The listing builds one solid part. Answer for the finished solid, in the listing's coordinates (mm). A direction names the side the tool comes from. Round coordinates to 2 decimals unless told otherwise and drop trailing zeros. Loops run counter-clockwise (first coordinate to the right, second up) from the corner with the lowest first, then second, coordinate; pieces in that order, holes last. Notation, with made-up numbers: (-33.75, 20.25) -> (24.25, 20.25) arc R12 cw to (24.25, 31.25) -> close; hole circle Ø7 at (-12, -1). An arc over 180 degrees is marked (long way). Write each question's results on one line, items separated by ' | '. Start each with the question number.
(1) The part is cut by section D-D (x = -9.75). Determine the outline of the cut face in (y, z), plus the area to 3 significant figures.
(2) The part is cut by section B-B (x = 0). Determine the outline of the cut face in (y, z).
(3) The part is cut by section C-C (z = 16.75). Determine the outline of the cut face in (x, y), plus the area to 3 significant figures.
(4) Straight lines are drawn through the part: probe 1 along Y at (x, z) = (0.25, 17.75); probe 2 along Z at (x, y) = (2.5, 5.25); probe 3 along Y at (x, z) = (-1.75, 25.25). For each, find the intervals that lie inside material, in ascending order.
(5) Flat-ended cylindrical pins translate along their axes: pin 1 (5 mm diameter, centred on x = -4, y = 5.5, fed in from +Z); pin 2 (1.5 mm diameter, centred on y = -13, z = 9, fed in from +X); pin 3 (10 mm diameter, centred on y = -1.5, z = 16, fed in from -X); pin 4 (6 mm diameter, centred on y = -8.5, z = 20, fed in from +X). Find the tip coordinate at first contact, or state that the pin passes through.
(6) The part is cut by section A-A (y = -4). Determine the outline of the cut face in (x, z), plus the area to 3 significant figures.
(7) Determine the mould class of faces 1 (the face through (-10.316, 3.91, 1.521)), 2 (the face through (-3, -7, 0)), 3 (the face through (11.693, -3.933, 1.479)) for opening direction Y: released by +Y, released by -Y, zero draft, split by the parting line, or undercut.
(8) For faces 4 (the face through (6, 2, 3)), 5 (the face through (0.33, 4.67, 1.48)), determine the directions among +Z, -Z, +X, -X, +Y, -Y from which every point of the face is accessible in a straight line to the end or side of a thin tool.
```python
from build123d import *

# Parameters (mm, degrees)
CROQUIS2_R            = 1.530907885
CORTAR_EXTRUIR1_DEPTH = 10


with BuildPart() as part:
    # Croquis1 → Revolución1 (revolve)
    with BuildSketch(Plane(origin=(0, 0, 0), x_dir=(0, 0, -1), z_dir=(1, 0, 0)), mode=Mode.PRIVATE) as revoluci_n1_sk:
        Polygon((0, 0), (0, 9), (-3, 9), (-3, 3), (-30, 3), (-30, 0), align=None)
    revolve(revoluci_n1_sk.sketch.rotate(Axis((0, -4, 49.046153846), (0, 0, -1)), 90), axis=Axis((0, -4, 49.046153846), (0, 0, -1)))

    # Croquis2 → Cortar-Extruir1 (cut)
    with BuildSketch(Plane(origin=(0, 0, 0), x_dir=(-1, 0, 0), z_dir=(0, 0, -1))):
        with Locations((0, 6.163841236)):
            Circle(CROQUIS2_R)
        with Locations((10.163841236, -4)):
            Circle(CROQUIS2_R)
        with Locations((0, -14.163841236)):
            Circle(CROQUIS2_R)
        with Locations((-10.163841236, -4)):
            Circle(CROQUIS2_R)
    extrude(amount=-CORTAR_EXTRUIR1_DEPTH, mode=Mode.SUBTRACT)


solid = part.part
```
Checked values:
1) outline: (-12.6, 0) -> (-5.47, 0) -> (-5.47, 3) -> (-12.6, 3) -> close; (-2.53, 0) -> (4.6, 0) -> (4.6, 3) -> (-2.53, 3) -> close | area: 42.7 mm2
2) outline: (-17, 0) -> (-15.69, 0) -> (-15.69, 3) -> (-17, 3) -> close; (-12.63, 0) -> (-8, 0) -> (-8, 30) -> (-11, 30) -> (-11, 3) -> (-12.63, 3) -> close; (0, 0) -> (4.63, 0) -> (4.63, 3) -> (3, 3) -> (3, 30) -> (0, 30) -> close; (7.69, 0) -> (9, 0) -> (9, 3) -> (7.69, 3) -> close
3) outline: circle Ø14 at (0, -4); hole circle Ø8 at (0, -4) | area: 104 mm2
4) probe 1: y = -11 to -7.99, -0.01 to 3 | probe 2: z = 0 to 3 | probe 3: y = -10.78 to -7.6, -0.4 to 2.78
5) pin 1: stops at z = 3 | pin 2: passes through | pin 3: stops at x = -7 | pin 4: stops at x = 6.84
6) outline: (-13, 0) -> (-11.69, 0) -> (-11.69, 3) -> (-13, 3) -> close; (-8.63, 0) -> (-4, 0) -> (-4, 30) -> (-7, 30) -> (-7, 3) -> (-8.63, 3) -> close; (4, 0) -> (8.63, 0) -> (8.63, 3) -> (7, 3) -> (7, 30) -> (4, 30) -> close; (11.69, 0) -> (13, 0) -> (13, 3) -> (11.69, 3) -> close | area: 198 mm2
7) face 1: split by the parting line | face 2: zero draft | face 3: undercut
8) face 4: +Z | face 5: +Z, -Z
